from build123d import *

# Parameters (mm, degrees)
F0_W     = 0.9482001415
F0_H     = 8.158806867
F0_R     = 2.5
F1_DEPTH = 1.5
F2_R     = 5
F3_R     = 5


with BuildPart() as f1:
    # F0 (on Top) → F1 (new body)
    with BuildSketch(Plane.XY):
        Polygon((-15, 20), (-60, 20), (-60, 0), (-15, 0), (0, 10), align=None)
        with BuildLine():
            add(Edge.make_bspline(
                [(-47.4459262549, 12.6766424166), (-46.3914776983, 11.62219386), (-46.3914776983, 9.7293649524)],
                knots=[0, 0, 0, 1, 1, 1], degree=2))
            add(Edge.make_bspline(
                [(-46.3914776983, 9.7293649524), (-46.3914776983, 7.7097522217), (-47.4878899146, 6.6410181639)],
                knots=[0, 0, 0, 1, 1, 1], degree=2))
            add(Edge.make_bspline(
                [(-47.4878899146, 6.6410181639), (-48.5843021309, 5.5722841062), (-50.6431999899, 5.5722841062)],
                knots=[0, 0, 0, 1, 1, 1], degree=2))
            Line((-50.6431999899, 5.5722841062), (-52.9038805532, 5.5722841062))
            Line((-52.9038805532, 5.5722841062), (-52.9038805532, 13.7310909731))
            Line((-52.9038805532, 13.7310909731), (-50.403917845, 13.7310909731))
            add(Edge.make_bspline(
                [(-50.403917845, 13.7310909731), (-48.5003748114, 13.7310909731), (-47.4459262549, 12.6766424166)],
                knots=[0, 0, 0, 1, 1, 1], degree=2))
        make_face(mode=Mode.SUBTRACT)
        with Locations((-44.0977619135, 9.6516875396)):
            Rectangle(F0_W, F0_H, mode=Mode.SUBTRACT)
        Polygon((-36.8380487777, 6.4204857393), (-36.8380487777, 5.5722841062), (-41.386195219, 5.5722841062), (-41.386195219, 13.7310909731), (-36.8380487777, 13.7310909731), (-36.8380487777, 12.8882464029), (-40.4379950775, 12.8882464029), (-40.4379950775, 10.259714184), (-37.0559026708, 10.259714184), (-37.0559026708, 9.4222266768), (-40.4379950775, 9.4222266768), (-40.4379950775, 6.4204857393), align=None, mode=Mode.SUBTRACT)
        Polygon((-32.5202560431, 12.8882464029), (-32.5202560431, 5.5722841062), (-33.4684561846, 5.5722841062), (-33.4684561846, 12.8882464029), (-36.0523462123, 12.8882464029), (-36.0523462123, 13.7310909731), (-29.9363660154, 13.7310909731), (-29.9363660154, 12.8882464029), align=None, mode=Mode.SUBTRACT)
        Polygon((-23.7632438138, 6.4311998652), (-23.7632438138, 5.5722841062), (-29.3720887184, 5.5722841062), (-29.3720887184, 6.315130168), (-25.0417961703, 12.877532277), (-29.2381621448, 12.877532277), (-29.2381621448, 13.7310909731), (-23.8864562616, 13.7310909731), (-23.8864562616, 12.9882449113), (-28.2167488097, 6.4311998652), align=None, mode=Mode.SUBTRACT)
        Polygon((-17.6365494911, 6.4204857393), (-17.6365494911, 5.5722841062), (-22.1846959324, 5.5722841062), (-22.1846959324, 13.7310909731), (-17.6365494911, 13.7310909731), (-17.6365494911, 12.8882464029), (-21.2364957909, 12.8882464029), (-21.2364957909, 10.259714184), (-17.8544033843, 10.259714184), (-17.8544033843, 9.4222266768), (-21.2364957909, 9.4222266768), (-21.2364957909, 6.4204857393), align=None, mode=Mode.SUBTRACT)
        with Locations((-11, 10)):
            Circle(F0_R, mode=Mode.SUBTRACT)
    extrude(amount=F1_DEPTH)

    # F2
    f2_edges = [f1.edges().sort_by_distance(p)[0] for p in [
        (0, 10, 0.75),
    ]]
    fillet(f2_edges, radius=F2_R)

    # F3
    f3_edges = [f1.edges().sort_by_distance(p)[0] for p in [
        (-60, 20, 0.75),
        (-60, 0, 0.75),
        (-15, 0, 0.75),
        (-15, 20, 0.75),
    ]]
    fillet(f3_edges, radius=F3_R)


solid = f1.part
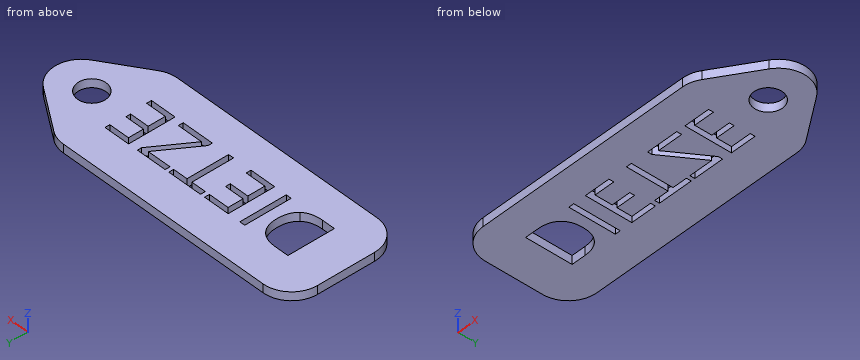
The listing builds one solid part. Answer for the finished solid, in the listing's coordinates (mm). Round coordinates to 2 decimals unless told otherwise and drop trailing zeros. Write each loop counter-clockwise with the first axis right and the second up, starting at its lowest first coordinate (ties: lowest second). Pieces come first, ordered by that corner, then holes. Notation, with made-up numbers: M 16.25,-32.75 L 57.25,-32.75 A15 ccw 57.25,-6.75 Z; hole C 39,35 d6. An arc over 180 degrees is marked long. Write each question's results on one line, items separated by ' | '. Start each with the question number.
(1) Find the intervals of material crossed by line 1 (Y direction, x = -37.5, z = 1.45); line 2 (Y direction, x = -31.5, z = 1.25); line 3 (Y direction, x = -44.5, z = 0.15), in increasing order.
(2) The part is cut by section C-C, the plane z = 1.25. Give the number of separate pieces and of enclosed holes in the cut face, and give its area (3 significant figures).
(3) The part is cut by section A-A, the plane x = -19. Write down the section's boundary in (y, z).
(4) The part is cut by section B-B, the plane x = -11. Write down the section's boundary in (y, z), and give its area (3 significant figures).
(5) This flat-tipped pin is pushed along its axis until it touches: P1, Ø0.7, axis at y = 13, z = 0.5, coming from the +X side. Where does it stop, or does it pass through?
(6) The part is cut by section D-D, the plane y = 16.5. Write down the section's boundary in (x, z), and give its area (3 significant figures).
Worked answers:
1) line 1: y = 0 to 5.57, 6.42 to 9.42, 10.26 to 12.89, 13.73 to 20 | line 2: y = 0 to 12.89, 13.73 to 20 | line 3: y = 0 to 5.57, 13.73 to 20
2) separate pieces: 1 | enclosed holes: 7 | area: 890 mm²
3) outline: M 0,0 L 5.57,0 L 5.57,1.5 L 0,1.5 Z; M 6.42,0 L 9.42,0 L 9.42,1.5 L 6.42,1.5 Z; M 10.26,0 L 12.89,0 L 12.89,1.5 L 10.26,1.5 Z; M 13.73,0 L 20,0 L 20,1.5 L 13.73,1.5 Z
4) outline: M 2.67,0 L 7.5,0 L 7.5,1.5 L 2.67,1.5 Z; M 12.5,0 L 17.33,0 L 17.33,1.5 L 12.5,1.5 Z | area: 14.5 mm²
5) P1: stops at x = -4.77
6) outline: M -59.77,0 L -9.75,0 L -9.75,1.5 L -59.77,1.5 Z | area: 75.0 mm²
